Part model, mm, in its own coordinate system. Coordinates: 2 decimals unless noted, no trailing zeros. Write each loop counter-clockwise with the first axis right and the second up, starting at its lowest first coordinate (ties: lowest second). Pieces come first, ordered by that corner, then holes. Notation, with made-up numbers: (30, 78) - (52, 78) arc R23 ccw to (52, 114) - close; hole circle Ø6 at (5.25, 80). An arc over 180 degrees is marked (long way). Use a Markdown table: item, result.
```python
from build123d import *

# Parameters (mm, degrees)
SKETCH1_W               = 63.5
SKETCH1_H               = 25.4
BOSS_EXTRUDE1_DEPTH     = 6.35
F_1_4_CLEARANCE_HOLE1_D = 6.7564
M3_CLEARANCE_HOLE1_D    = 3.4


with BuildPart() as part:
    # Sketch1 → Boss-Extrude1 (new body)
    with BuildSketch(Plane.XY):
        with Locations((31.75, 12.7)):
            Rectangle(SKETCH1_W, SKETCH1_H)
    extrude(amount=BOSS_EXTRUDE1_DEPTH)

    # 1/4 Clearance Hole1 (through all)
    with Locations(Plane.XY.offset(6.35)):
        with Locations((12.7, 6.35), (12.7, 19.05)):
            Hole(F_1_4_CLEARANCE_HOLE1_D / 2)

    # M3 Clearance Hole1 (through all)
    with Locations(Plane.XY.offset(6.35)):
        with Locations((50.8, 12.7)):
            Hole(M3_CLEARANCE_HOLE1_D / 2)


solid = part.part
```
Item 1: Band-saw the part on C-C, the plane z = 5. Give the cut face in (x, y), then the cut area to 3 significant figures.
From the geometry:
| item | result |
|---|---|
| outline | (0, 0) - (63.5, 0) - (63.5, 25.4) - (0, 25.4) - close; hole circle Ø6.76 at (12.7, 6.35); hole circle Ø6.76 at (12.7, 19.05); hole circle Ø3.4 at (50.8, 12.7) |
| area | 1,530 mm^2 |
Item 2: Drill centre lines: probe 1 along Y at (x, z) = (12.7, 4.75); probe 2 along Y at (x, z) = (50.8, 4.75); probe 3 along X at (y, z) = (4.5, 5.25). Where is each one in solid material? Low to high.
From the geometry:
| item | result |
|---|---|
| probe 1 | 0 to 2.97, 9.73 to 15.67, 22.43 to 25.4 |
| probe 2 | 0 to 11, 14.4 to 25.4 |
| probe 3 | 0 to 9.87, 15.53 to 63.5 |
Item 3: Drop a flat-ended pin along its axis: P1, Ø2.5, axis at x = 50.8, y = 12.7, coming from the -Z side. Give the stop position or say it passes through.
From the geometry:
| item | result |
|---|---|
| P1 | through |
Item 4: Two-plate mould, pull along Y, no slides. Class faces 1 (the face through (13.43, 15.75, 3.13)), 2 (the face through (31, 25.4, 3)), 3 (the face through (0, 13, 3)), 4 (the face through (31, 0, 3)): pulls with the +Y half, pulls with the -Y half, needs draft (parallel to the pull), parting line crosses it, or undercut.
From the geometry:
| item | result |
|---|---|
| face 1 | undercut |
| face 2 | pulls with the +Y half |
| face 3 | needs draft |
| face 4 | pulls with the -Y half |
Item 5: Band-saw the part on A-A, the plane y = 19.05. Give the cut face in (x, z), then the cut area to 3 significant figures.
From the geometry:
| item | result |
|---|---|
| outline | (0, 0) - (9.32, 0) - (9.32, 6.35) - (0, 6.35) - close; (16.08, 0) - (63.5, 0) - (63.5, 6.35) - (16.08, 6.35) - close |
| area | 360 mm^2 |
Item 6: Band-saw the part on D-D, the plane x = 12.7. Give the cut face in (y, z), then the cut area to 3 significant figures.
From the geometry:
| item | result |
|---|---|
| outline | (0, 0) - (2.97, 0) - (2.97, 6.35) - (0, 6.35) - close; (9.73, 0) - (15.67, 0) - (15.67, 6.35) - (9.73, 6.35) - close; (22.43, 0) - (25.4, 0) - (25.4, 6.35) - (22.43, 6.35) - close |
| area | 75.5 mm^2 |
Item 7: Band-saw the part on B-B, the plane x = 50.8. Give the cut face in (y, z), then the cut area to 3 significant figures.
From the geometry:
| item | result |
|---|---|
| outline | (0, 0) - (11, 0) - (11, 6.35) - (0, 6.35) - close; (14.4, 0) - (25.4, 0) - (25.4, 6.35) - (14.4, 6.35) - close |
| area | 140 mm^2 |
